For this review, take the finished solid that the model builds, in its own axes (mm). A direction names the side the tool comes from. Round coordinates to 2 decimals unless told otherwise and drop trailing zeros. Order: outer loops, then holes, each group sorted by start corner. A loop starts at its lowest first (then second) coordinate and runs counter-clockwise, first axis right, second up. Notation, with made-up numbers: (53, -28) -> (89, -28) arc R20 ccw to (89, -11) -> close; hole circle Ø5 at (49, -39). An arc over 180 degrees is marked (long way). Use a Markdown table: item, result. Add a question column.
1) Draft analysis for pull direction X (two halves, no side actions). For faces 1 (the face through (10, -25, 2)), 2 (the face through (-16, -3, 2)), 3 (the face through (-7, -10, 0)), 4 (the face through (5, -25, 2)), state which applies: pulls with the +X half, pulls with the -X half, needs draft (parallel to the pull), parting line crosses it, or undercut.
2) Wall thickness on line 1 along Y through (x, z) = (0, 3.2); line 2 along X through (y, z) = (5, 3.8); line 3 along Y through (x, z) = (11.5, 2.2): over which ranges is each line inside the solid? List them lowest first. Write a range as [from, to].
3) Consider section C-C (z = 4.1). State the section outline as (x, y) points, plus the area to 3 significant figures.
4) Machinability: for faces 5 (the face through (13, -22, 2)), 6 (the face through (-5, -25, 2)), 7 (the face through (-13, -22, 2)), which of the approach directions +Z, -Z, +X, -X, +Y, -Y give a long, thin tool a straight path to every point of the face, cutting with its end or side? Answer none if there is none.
5) Consider section B-B (x = 0). State the section outline as (y, z) points.
6) Clearance check with flat-ended pins moving along their axes: P1, Ø1.5, axis at y = -24, z = 2.5, coming from the +X side; P2, Ø1, axis at x = -0.5, z = 4.5, coming from the -Y side. State where each tip first meets the part, or that it passes through.
7) Consider section A-A (y = 0). State the section outline as (x, z) points.
```python
from build123d import *

# Parameters (mm, degrees)
SKETCH1_W           = 5
SKETCH1_H           = 5
SKETCH1_W_2         = 32
SKETCH1_H_2         = 38
SKETCH1_R           = 11
BOSS_EXTRUDE1_DEPTH = 5


with BuildPart() as part:
    # Sketch1 → Boss-Extrude1 (new body)
    # profile 1 of 3: a face of its own
    with BuildSketch(Plane.XY):
        with Locations((7.5, -24.5)):
            Rectangle(SKETCH1_W, SKETCH1_H)
    # profile 2 of 3: a face of its own
    with BuildSketch(Plane.XY):
        with Locations((-7.5, -24.5)):
            Rectangle(SKETCH1_W, SKETCH1_H)
    # profile 3 of 3: a face of its own
    with BuildSketch(Plane.XY):
        with Locations((0, -3)):
            Rectangle(SKETCH1_W_2, SKETCH1_H_2)
        Circle(SKETCH1_R, mode=Mode.SUBTRACT)
    extrude(amount=BOSS_EXTRUDE1_DEPTH)


solid = part.part
```
Results list:
| question | item | result |
|---|---|---|
| 1 | face 1 | pulls with the +X half |
| 1 | face 2 | pulls with the -X half |
| 1 | face 3 | needs draft |
| 1 | face 4 | undercut |
| 2 | line 1 | [-22, -11], [11, 16] |
| 2 | line 2 | [-16, -9.8], [9.8, 16] |
| 2 | line 3 | [-22, 16] |
| 3 | outline | (-16, -22) -> (-10, -22) -> (-10, -27) -> (-5, -27) -> (-5, -22) -> (5, -22) -> (5, -27) -> (10, -27) -> (10, -22) -> (16, -22) -> (16, 16) -> (-16, 16) -> close; hole circle Ø22 at (0, 0) |
| 3 | area | 886 mm2 |
| 4 | face 5 | +Z, -Z, +X, -Y |
| 4 | face 6 | +Z, -Z, -Y |
| 4 | face 7 | +Z, -Z, -X, -Y |
| 5 | outline | (-22, 0) -> (-11, 0) -> (-11, 5) -> (-22, 5) -> close; (11, 0) -> (16, 0) -> (16, 5) -> (11, 5) -> close |
| 6 | P1 | x = 10 |
| 6 | P2 | y = -22 |
| 7 | outline | (-16, 0) -> (-11, 0) -> (-11, 5) -> (-16, 5) -> close; (11, 0) -> (16, 0) -> (16, 5) -> (11, 5) -> close |
